Model file for the job. Use its own axes, mm. A direction names the side the tool comes from. Give positions to 0.01 mm unless a question says otherwise; leave off trailing zeros. Loops run counter-clockwise (first coordinate to the right, second up) from the corner with the lowest first, then second, coordinate; pieces in that order, holes last. Notation, with made-up numbers: M 78,-25 L 119,-25 A26 ccw 119,-5 Z; hole C 13,-24 d8. An arc over 180 degrees is marked long. Answer in a Markdown table with one row per item.
```python
from build123d import *

# Parameters (mm, degrees)
F0_R      = 7.0358
F1_DEPTH  = 1.524
F2_R      = 6.2357
F4_R      = 6.0071
F5_FACE_R = 6.0071
F7_R      = 4.1783
F9_DEPTH  = 6.223


with BuildPart() as f1:
    # F0 (on Top) → F1 (new body)
    with BuildSketch(Plane.XY):
        Circle(F0_R)
    extrude(amount=F1_DEPTH)

    # F2 (on face) → F5 section 0
    with BuildSketch(Plane.XY.offset(1.524)):
        Circle(F2_R)
    # F4 (on offset) → F5 section 1
    with BuildSketch(Plane.XY.offset(39.5732)):
        Circle(F4_R)
    loft()

    # F5_face (on face) → F8 section 0
    with BuildSketch(Plane.XY.offset(39.5732)):
        Circle(F5_FACE_R)
    # F7 (on offset) → F8 section 1
    with BuildSketch(Plane.XY.offset(52.197)):
        Circle(F7_R)
    loft()

    # F9 (add): a face of the model
    f9_faces = [f1.faces().sort_by_distance(p)[0] for p in [
        (0, 0, 52.197),
    ]]
    extrude(f9_faces, amount=F9_DEPTH)


solid = f1.part
```
(1) Which spindle directions (+Z, -Z, +X, -X, +Y, -Y) get a long thin tool onto all of the face, cutting with end or side? Do faces 4 (the conical face through (-0.797, 6.068, 20.815)), 5 (the flat face through (0, 0, 58.42)). Say none if no direction does.
Established:
| item | result |
|---|---|
| face 4 | +Z |
| face 5 | +Z, +X, -X, +Y, -Y |
(2) Flat gauge pins, fed straight in: P1, Ø2, axis at y = 1, z = 21.5, coming from the +X side; P2, Ø2, axis at y = -4.5, z = 20.5, coming from the +X side; P3, Ø3, axis at y = -4, z = 18.5, coming from the -X side. Where does each tip first touch, or does it go through?
Established:
| item | result |
|---|---|
| P1 | stops at x = 6.12 |
| P2 | stops at x = 5.02 |
| P3 | stops at x = -5.6 |
(3) Wall check: L1, parallel to Y at x = 1.5, z = 8.5; L2, parallel to X at y = 1.5, z = 10; L3, parallel to Z at x = 6, y = 2. Give the ranges that are in metal, low to high.
Established:
| item | result |
|---|---|
| L1 | y = -6.01 to 6.01 |
| L2 | x = -6 to 6 |
| L3 | z = 0 to 1.52 |
(4) Mould opens along Z. For faces 1 (the cylindrical face through (-0.916, 6.976, 0.751)), 2 (the flat face through (-4, -5, 1.524)), 3 (the flat face through (0, 0, 0)) say: pulls with the +Z half, pulls with the -Z half, needs draft (parallel to the pull), parting line crosses it, or undercut.
Established:
| item | result |
|---|---|
| face 1 | needs draft |
| face 2 | pulls with the +Z half |
| face 3 | pulls with the -Z half |
(5) Saw through at A-A, the plane z = 13.5. Give the cut face in (x, y), and give its area (3 significant figures).
Established:
| item | result |
|---|---|
| outline | C 0,0 d12.33 |
| area | 119 mm2 |
(6) Saw through at B-B, the plane z = 23. Give the cut face in (x, y), and give its area (3 significant figures).
Established:
| item | result |
|---|---|
| outline | C 0,0 d12.21 |
| area | 117 mm2 |
